from build123d import *

# Parameters (mm, degrees)
BOSS_EXTRUDE5_OUTLINE_R = 42.5
BOSS_EXTRUDE5_DEPTH     = 22
SKETCH11_W              = 23
SKETCH11_H              = 20
BOSS_EXTRUDE6_DEPTH     = 22
SKETCH12_W              = 23
SKETCH12_H              = 20
CUT_EXTRUDE1_DEPTH      = 19.5
SKETCH13_W              = 20
SKETCH13_H              = 18
CUT_EXTRUDE2_DEPTH      = 39


# Read off the part's stored shape, not the designer's step: Boss-Extrude5
with BuildPart() as part:
    # Boss-Extrude5 outline → Boss-Extrude5 (new body)
    with BuildSketch(Plane(origin=(0, 25, 0), x_dir=(1, 0, 0), z_dir=(0, 1, 0))):
        Circle(BOSS_EXTRUDE5_OUTLINE_R)
    extrude(amount=BOSS_EXTRUDE5_DEPTH)

    # Sketch11 → Boss-Extrude6 (add, symmetric)
    with BuildSketch(Plane(origin=(0, 47, 0), x_dir=(1, 0, 0), z_dir=(0, 1, 0))):
        with Locations((-0.729469309, 47.32480688)):
            Rectangle(SKETCH11_W, SKETCH11_H)
    extrude(amount=BOSS_EXTRUDE6_DEPTH, both=True)

    # Sketch12 → Cut-Extrude1 (cut, symmetric)
    with BuildSketch(Plane(origin=(0, 69, 0), x_dir=(1, 0, 0), z_dir=(0, 1, 0))):
        with Locations((-0.729469309, 47.32480688)):
            Rectangle(SKETCH12_W, SKETCH12_H)
    extrude(amount=CUT_EXTRUDE1_DEPTH, both=True, mode=Mode.SUBTRACT)

    # Sketch13 → Cut-Extrude2 (cut)
    with BuildSketch(Plane(origin=(0, 49.5, 0), x_dir=(1, 0, 0), z_dir=(0, 1, 0))):
        with Locations((-0.729469309, 48.32480688)):
            Rectangle(SKETCH13_W, SKETCH13_H)
    extrude(amount=-CUT_EXTRUDE2_DEPTH, mode=Mode.SUBTRACT)


solid = part.part
Can you work these out from the model? Positions are in its coordinate system, mm. A direction names the side the tool comes from. Coordinates: 2 decimals unless noted, no trailing zeros. Order: outer loops, then holes, each group sorted by start corner. A loop starts at its lowest first (then second) coordinate and runs counter-clockwise, first axis right, second up. Notation, with made-up numbers: M 39.5,53 L 66.5,53 A33 ccw 66.5,88 Z; hole C 27.25,26.25 d4. An arc over 180 degrees is marked long. Answer as CSV lines item,"result".
(1) On a 3-axis mill with a long thin cutter (end or side, diameter ignored), from which of +Z, -Z, +X, -X, +Y, -Y can I reach the whole of each face in a straight line? I mean faces 5 (the cylindrical face through (-0.95, 35.85, 42.49)), 6 (the flat face through (-10.729, 37, -48)). Say none if no direction works.
Geometry check:
face 5,"+Y, -Y"
face 6,"-Z, +Y, -Y"
(2) Suppose I cut it at D-D on x = 27. Please give me the cut outline in (y, z), plus the area to 3 significant figures.
Geometry check:
outline,"M 25,-32.82 L 47,-32.82 L 47,32.82 L 25,32.82 Z"
area,"1,440 mm^2"
(3) If we mould it in two halves opening along X, with no side actions, what happens to faces 1 (the flat face through (-1, 37, -39.325)), 2 (the flat face through (9.271, 37, -48)), 3 (the flat face through (-1, 48, -37.325)), 4 (the flat face through (10.771, 37, -49))? For each: released by +X, released by -X, zero draft, split by the parting line, or undercut.
Geometry check:
face 1,"undercut"
face 2,"undercut"
face 3,"zero draft"
face 4,"released by +X"
(4) Suppose I cut it at B-B on x = 0. Please give me the cut outline in (y, z).
Geometry check:
outline,"M 25,-39.32 L 49.5,-39.32 L 49.5,-37.32 L 47,-37.32 L 47,42.5 L 25,42.5 Z"
(5) Please list where these lines run through material, in increasing order: L1, parallel to Y at x = -25, z = -2.5; L2, parallel to Z at x = -12, y = 46; L3, parallel to Z at x = -33.5, y = 36.25.
Geometry check:
L1,"25 to 47"
L2,"-57.32 to 40.77"
L3,"-26.15 to 26.15"
(6) Suppose I cut it at A-A on z = 0. Please give me the cut outline in (x, y).
Geometry check:
outline,"M -42.5,25 L 42.5,25 L 42.5,47 L -42.5,47 Z"
(7) Suppose I cut it at C-C on y = 30.25. Please give me the cut outline in (x, z).
Geometry check:
outline,"M -12.23,-57.32 L -10.73,-57.32 L -10.73,-39.32 L 9.27,-39.32 L 9.27,-57.32 L 10.77,-57.32 L 10.77,-41.11 A42.5 ccw long -12.23,-40.7 Z"
(8) I'm going to push flat-ended pins straight in: pin 1 (1.5 mm diameter, centred on x = 30, z = 9.5, fed in from +Y); pin 2 (3 mm diameter, centred on y = 32.5, z = 5, fed in from +X); pin 3 (2 mm diameter, centred on y = 39.5, z = -10.5, fed in from -X). Where does each tip first touch, or does it pass through?
Geometry check:
pin 1,"y = 47"
pin 2,"x = 42.36"
pin 3,"x = -41.42"
